Read the model definition and answer for the solid it produces. Units are mm, in the model's axes. A direction names the side the tool comes from. Give positions to 0.01 mm unless a question says otherwise; leave off trailing zeros. Loops run counter-clockwise (first coordinate to the right, second up) from the corner with the lowest first, then second, coordinate; pieces in that order, holes last. Notation, with made-up numbers: (76, -11.75) -> (94, -11.75) arc R20 cw to (94, -2.75) -> close; hole circle Ø3 at (39.25, 66). An arc over 180 degrees is marked (long way). Return JSON: item names as keys, results as strings. Group by question number.
from build123d import *

# Parameters (mm, degrees)
SKETCH008_W         = 79.607547
SKETCH008_H         = 84.957516
PAD002_DEPTH        = 20
SKETCH009_W         = 73.187564
SKETCH009_H         = 77.253553
POCKET004_DEPTH     = 14
REVOLUTION_ANGLE    = -180
SKETCH001_W         = 35
SKETCH001_H         = 1.5
PAD_DEPTH           = 1
SKETCH002_W         = 35
SKETCH002_H         = 1.5
POCKET_DEPTH        = 1
SKETCH003_R         = 4
PAD001_DEPTH        = 8
SKETCH004_W         = 1
SKETCH004_H         = 9.534319
REVOLUTION001_ANGLE = -180
SKETCH005_R         = 1
POCKET001_DEPTH     = 7
SKETCH006_R         = 2.5
POCKET002_DEPTH     = 10
POCKET003_DEPTH     = 10


with BuildPart() as body001:
    # Sketch008 → Pad002 (new body)
    with BuildSketch(Plane.XY):
        with Locations((46.254125, -8.464853)):
            Rectangle(SKETCH008_W, SKETCH008_H)
    extrude(amount=PAD002_DEPTH)

    # Sketch009 → Pocket004 (cut)
    with BuildSketch(Plane.XY):
        with Locations((46.664473, -8.115113)):
            Rectangle(SKETCH009_W, SKETCH009_H)
    extrude(amount=POCKET004_DEPTH, mode=Mode.SUBTRACT)


with BuildPart() as body001_1:
    # Body001 placement: moved
    add(body001.part.moved(Location((0, 34, 0))))


with BuildPart() as fusion:
    # Sketch → Revolution (revolve)
    with BuildSketch(Plane.XY):
        with BuildLine():
            Line((-35, -17), (35, -17))
            ThreePointArc((35, -17), (46.543396, -15.207817), (57, -10))
            Line((57, -10), (52, -10))
            Line((52, -10), (52, -7.5))
            Line((52, -7.5), (50, -7.5))
            Line((50, -7.5), (50, -11.758585))
            ThreePointArc((48, -12.600664), (49.00633, -12.194658), (50, -11.758585))
            Line((48, -9.5), (48, -12.600664))
            Line((35, -9.5), (48, -9.5))
            Line((35, -14), (35, -9.5))
            Line((35, -14), (-35, -14))
            Line((-35, -14), (-35, -9.5))
            Line((-35, -9.5), (-48, -9.5))
            Line((-48, -9.5), (-48, -12.600664))
            ThreePointArc((-50, -11.758585), (-49.00633, -12.194658), (-48, -12.600664))
            Line((-50, -11.758585), (-50, -7.5))
            Line((-50, -7.5), (-52, -7.5))
            Line((-52, -7.5), (-52, -10))
            Line((-52, -10), (-57, -10))
            ThreePointArc((-57, -10), (-46.543396, -15.207817), (-35, -17))
        make_face()
    revolve(axis=Axis((0, 0, 0), (1, 0, 0)), revolution_arc=REVOLUTION_ANGLE)

    # Sketch001 → Pad (new body)
    with BuildSketch(Plane.XY):
        with Locations((17.5, 14.75)):
            Rectangle(SKETCH001_W, SKETCH001_H)
    pad = extrude(amount=-PAD_DEPTH)

    # Mirrored: Pad across XZ
    add(pad.mirror(Plane.XZ))

    # Sketch002 → Pocket (cut)
    with BuildSketch(Plane.XY):
        with Locations((-17.5, 14.75)):
            Rectangle(SKETCH002_W, SKETCH002_H)
    pocket = extrude(amount=POCKET_DEPTH, mode=Mode.SUBTRACT)

    # Mirrored001: Pocket across XZ
    add(pocket.mirror(Plane.XZ), mode=Mode.SUBTRACT)

    # Sketch003 → Pad001 (join)
    with BuildSketch(Plane.XY):
        with Locations((43, -8)):
            Circle(SKETCH003_R)
        with Locations((-43, -8)):
            Circle(SKETCH003_R)
        with Locations((-43, 8)):
            Circle(SKETCH003_R)
        with Locations((43, 8)):
            Circle(SKETCH003_R)
    extrude(amount=PAD001_DEPTH)

    # Sketch004 → Revolution001 (revolve)
    with BuildSketch(Plane.XY):
        with Locations((43, -7.767159)):
            Rectangle(SKETCH004_W, SKETCH004_H)
    revolution001 = revolve(axis=Axis((0, 0, 0), (1, 0, 0)), revolution_arc=REVOLUTION001_ANGLE)

    # Mirrored002: Revolution001 across YZ
    add(revolution001.mirror(Plane.YZ))

    # Sketch005 → Pocket001 (cut)
    with BuildSketch(Plane.XY):
        with Locations((43, 8)):
            Circle(SKETCH005_R)
        with Locations((43, -8)):
            Circle(SKETCH005_R)
    extrude(amount=POCKET001_DEPTH, mode=Mode.SUBTRACT)

    # Sketch006 → Pocket002 (cut)
    with BuildSketch(Plane.XY):
        with Locations((-43, 8)):
            Circle(SKETCH006_R)
        with Locations((-43, -8)):
            Circle(SKETCH006_R)
    extrude(amount=POCKET002_DEPTH, mode=Mode.SUBTRACT)

    # Sketch007 → Pocket003 (cut)
    with BuildSketch(Plane.XY.offset(20)):
        with BuildLine():
            ThreePointArc((-39.5, 8), (-43, 11.5), (-46.5, 8))
            Line((-46.5, 8), (-46.5, -8))
            ThreePointArc((-46.5, -8), (-43, -11.5), (-39.5, -8))
            Line((-39.5, 8), (-39.5, -8))
        make_face()
    extrude(amount=-POCKET003_DEPTH, mode=Mode.SUBTRACT)

    # Fusion: union Body001
    add(body001_1.part)


solid = fusion.part
1. Determine the mould class of faces 5 (the cylindrical face through (-15, 0, 14)), 6 (the flat face through (54, -12.742, 8)), 7 (the flat face through (83.258, 25, 7)), 8 (the flat face through (10.071, -12, 13)) for opening direction Z: pulls with the +Z half, pulls with the -Z half, needs draft (parallel to the pull), parting line crosses it, or undercut.
2. Section A-A on x = 24.5 is taken. Determine the outline of the cut face in (y, z), then the cut area to 3 significant figures.
3. Flat-ended cylindrical pins translate along their axes: pin 1 Ø12 at (x, z) = (-36.5, 6.5) entering from -Y; pin 2 Ø10.5 at (y, z) = (-1.5, 4) entering from -X; pin 3 Ø0.5 at (y, z) = (15, -0.5) entering from +X; pin 4 Ø7 at (y, z) = (5.5, 4.5) entering from -X. Find the tip coordinate at first contact, or state that the pin passes through.
4. Straight lines are drawn through the part: line 1 (Z direction, x = 49, y = 36); line 2 (Y direction, x = 43, z = 4.75); line 3 (Z direction, x = 43.5, y = 6). For each, find the intervals that lie inside material, in ascending order. Write a range as from..to.
5. Which of the six approach directions +Z, -Z, +X, -X, +Y, -Y give full straight-line access (tool end or side, diameter ignored) to faces 1 (the flat face through (-43, 0, 10)), 2 (the flat face through (35, 1, 10)), 3 (the cylindrical face through (23, 15, 8)), 4 (the flat face through (-52, 0, 8))?
6. Section B-B on y = 54 is taken. Determine the outline of the cut face in (x, z).
Completed:
{
 "1": {"face 5": "pulls with the -Z half", "face 6": "undercut", "face 7": "needs draft", "face 8": "undercut"},
 "2": {"outline": "(-17, 0) -> (-15.5, 0) -> (-15.5, -1) -> (-14, -1) -> (-14, 0) -> (-12.74, 0) -> (-12.74, 5.8) arc R14 cw to (14, 0) -> (14, -1) -> (15.5, -1) -> (15.5, 0) -> (17, 0) arc R17 ccw to (9.64, 14) -> (64.51, 14) -> (64.51, 0) -> (68.01, 0) -> (68.01, 20) -> (-16.94, 20) -> (-16.94, 1.38) arc R17 ccw to start; hole (-12.74, 11.25) arc R17 cw to (-9.64, 14) -> (-12.74, 14) -> close", "area": "699 mm²"},
 "3": {"pin 1": "stops at y = -16.99", "pin 2": "stops at x = -52", "pin 3": "stops at x = 35", "pin 4": "stops at x = -57"},
 "4": {"line 1": "z = 14..20", "line 2": "y = -16.94..-9, -7..7, 9..15.44, 64.51..68.01", "line 3": "z = 0..20"},
 "5": {"face 1": "+Z", "face 2": "-Z", "face 3": "none", "face 4": "-Z, -X"},
 "6": {"outline": "(6.45, 0) -> (10.07, 0) -> (10.07, 14) -> (83.26, 14) -> (83.26, 0) -> (86.06, 0) -> (86.06, 20) -> (6.45, 20) -> close"}
}
